Job drawing, mm, ordinate dimensions from the low corner. One solid piece. Coordinates: 2 decimals unless noted, no trailing zeros. Write each loop counter-clockwise with the first axis right and the second up, starting at its lowest first coordinate (ties: lowest second). Pieces come first, ordered by that corner, then holes.
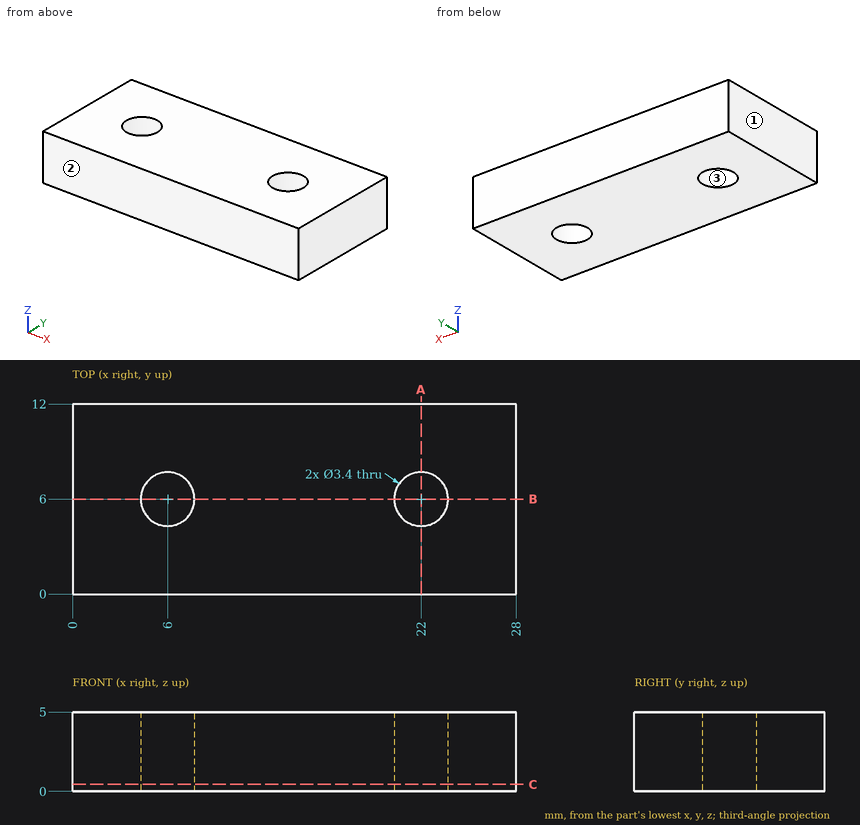
1. Probe line 1 along Y through (x, z) = (22, 3.4); line 2 along X through (y, z) = (5, 2.4); line 3 along X through (y, z) = (4.75, 0.8). List the from-to ranges inside material, lowest first.
Computed values:
line 1: y = 0 to 4.3, 7.7 to 12
line 2: x = 0 to 4.63, 7.37 to 20.63, 23.37 to 28
line 3: x = 0 to 4.85, 7.15 to 20.85, 23.15 to 28
2. Mould opens along X. For the marked faces 1, 2 and 3 say: +X half, -X half, draft (parallel to the pull), parting line (faces both ways), or undercut.
Computed values:
face 1: -X half
face 2: draft
face 3: undercut
3. Saw through at C-C on z = 0.45. List the corners of the cut face in (x, y).
Computed values:
outline: (0, 0) - (28, 0) - (28, 12) - (0, 12) - close; hole circle Ø3.4 at (6, 6); hole circle Ø3.4 at (22, 6)
4. Saw through at A-A on x = 22. List the corners of the cut face in (y, z), plus the area to 3 significant figures.
Computed values:
outline: (0, 0) - (4.3, 0) - (4.3, 5) - (0, 5) - close; (7.7, 0) - (12, 0) - (12, 5) - (7.7, 5) - close
area: 43.0 mm2
5. Saw through at B-B on y = 6. List the corners of the cut face in (x, z), plus the area to 3 significant figures.
Computed values:
outline: (0, 0) - (4.3, 0) - (4.3, 5) - (0, 5) - close; (7.7, 0) - (20.3, 0) - (20.3, 5) - (7.7, 5) - close; (23.7, 0) - (28, 0) - (28, 5) - (23.7, 5) - close
area: 106 mm2
6. Flat gauge pin, fed straight in: pin 1 (4.5 mm diameter, centred on x = 6, y = 6, fed in from -Z). Where does the tip first touch, or does it go through?
Computed values:
pin 1: stops at z = 0
